```python
from build123d import *

# Parameters (mm, degrees)
F0_W     = 1
F0_H     = 2.4
F1_DEPTH = 10


# Not quite as in the source:
# - a feature names something its author has since deleted; it is built from what else it names


with BuildPart() as f1:
    # F0 (on Top) → F1 (new body)
    with BuildSketch(Plane.XY):
        with Locations((10.9311291858, -6.7)):
            Rectangle(F0_W, F0_H)
        with Locations((-10.6688708142, -6.7)):
            Rectangle(F0_W, F0_H)
        Polygon((-2.45, -8.5), (-2.45, -7.9), (-3.85, -7.9), (-1.45, -10.5), (-1.45, -8.5), align=None)
        with BuildLine():
            Line((-11.1688708142, -5.5), (-10.1688708142, -5.5))
            Line((-10.1688708142, -5.5), (-10.1688708142, -4.6410811281))
            ThreePointArc((-10.1688708142, -4.6410811281), (-10.8661281522, -4.8408828578), (-11.1688708142, -5.5))
        make_face()
        with BuildLine():
            Line((10.4311291858, -4.5), (10.4311291858, -5.5))
            Line((10.4311291858, -5.5), (11.4311291858, -5.5))
            ThreePointArc((11.4311291858, -5.5), (11.1382359669, -4.7928932188), (10.4311291858, -4.5))
        make_face()
        Polygon((-1.45, -5.5), (-2.45, -5.5), (-2.45, -7.9), (-2.45, -8.5), (-1.45, -8.5), align=None)
        Polygon((2.45, -5.5), (1.45, -5.5), (1.45, -8.5), (2.45, -8.5), (2.45, -7.9), align=None)
        with BuildLine():
            Line((-10.1688708142, -4.6410811281), (-10.1688708142, -5.5))
            Line((-10.1688708142, -5.5), (-2.45, -5.5))
            Line((-2.45, -5.5), (-1.45, -5.5))
            Line((-1.45, -5.5), (1.45, -5.5))
            Line((1.45, -5.5), (2.45, -5.5))
            Line((2.45, -5.5), (10.4311291858, -5.5))
            Line((10.4311291858, -5.5), (10.4311291858, -4.5))
            Line((10.4311291858, -4.5), (8.1, -4.5))
            ThreePointArc((8.1, -4.5), (4.5644660941, -3.0355339059), (3.1, 0.5))
            Line((3.1, 0.5), (3.1, 4))
            ThreePointArc((3.1, 4), (2.6606601718, 5.0606601718), (1.6, 5.5))
            Line((1.6, 5.5), (1.1, 5.5))
            Line((1.1, 5.5), (1.1, -4))
            Line((1.1, -4), (-1.1, -4))
            Line((-1.1, -4), (-1.1, 5.5))
            Line((-1.1, 5.5), (-1.6, 5.5))
            ThreePointArc((-1.6, 5.5), (-2.6606601718, 5.0606601718), (-3.1, 4))
            Line((-3.1, 4), (-3.1, 0.3589188719))
            ThreePointArc((-3.1, 0.3589188719), (-4.5644660941, -3.176615034), (-8.1, -4.6410811281))
            Line((-8.1, -4.6410811281), (-10.1688708142, -4.6410811281))
        make_face()
        Polygon((2.45, -8.5), (1.45, -8.5), (1.45, -10.5), (3.85, -7.9), (2.45, -7.9), align=None)
    extrude(amount=F1_DEPTH)


solid = f1.part
```
Source: CAD feature listing. Evaluate the final solid. Frame: model axes, mm. A direction names the side the tool comes from. Round coordinates to 2 decimals unless told otherwise and drop trailing zeros. Loops run counter-clockwise (first coordinate to the right, second up) from the corner with the lowest first, then second, coordinate; pieces in that order, holes last.
1. Contact query for flat-ended pins moving along their axis: pin 1 (1.9 mm diameter, centred on x = 9, z = 3, fed in from +Y); pin 2 (1.8 mm diameter, centred on y = 1.5, z = 3, fed in from -X); pin 3 (6 mm diameter, centred on x = 6.5, z = 1.5, fed in from +Y). Output: stop coordinate, or through.
2. Mould query, pull axis X, two halves, no side actions, for faces 6 (the flat face through (-1.45, -8, 5)), 7 (the flat face through (-11, -7.9, 5)), 8 (the cylindrical face through (4.6, -3.07, 4.93)). Classes: released by +X, released by -X, zero draft, split by the parting line, or undercut.
3. Section query A-A on y = 2. Output: boundary loops of the cut face in (x, z).
4. Ray query, L1, parallel to X at y = -5.75, z = 9.5; L2, parallel to X at y = 0.25, z = 5.5; L3, parallel to Y at x = 0.5, z = 3. Return the intervals inside material, ascending.
5. Section query C-C on x = -0.5. Output: boundary loops of the cut face in (y, z).
6. Section query D-D on y = -3.75. Output: boundary loops of the cut face in (x, z).
7. Access query for faces 1 (the flat face through (-2.45, -7, 5)), 2 (the flat face through (9, -4.5, 5)), 3 (the flat face through (11, -7.9, 5)), 4 (the flat face through (1.1, 1, 5)), 5 (the flat face through (10.431, -7, 5)). Directions: +Z, -Z, +X, -X, +Y, -Y. A direction counts if a zero-diameter tool reaches every point of the face in a straight line with its end or side. Return the directions, or none.
Answers below:
1. pin 1: stops at y = -4.5
1. pin 2: stops at x = -3.1
1. pin 3: stops at y = -1.46
2. face 6: undercut
2. face 7: zero draft
2. face 8: released by +X
3. outline: (-3.1, 0) - (-1.1, 0) - (-1.1, 10) - (-3.1, 10) - close; (1.1, 0) - (3.1, 0) - (3.1, 10) - (1.1, 10) - close
4. L1: x = -11.17 to -10.17, -2.45 to -1.45, 1.45 to 2.45, 10.43 to 11.43
4. L2: x = -3.1 to -1.1, 1.1 to 3.11
4. L3: y = -5.5 to -4
5. outline: (-5.5, 0) - (-4, 0) - (-4, 10) - (-5.5, 10) - close
6. outline: (-5.25, 0) - (-1.1, 0) - (-1.1, 10) - (-5.25, 10) - close; (1.1, 0) - (5.47, 0) - (5.47, 10) - (1.1, 10) - close
7. face 1: +Z, -Z
7. face 2: +Z, -Z, +X, +Y
7. face 3: +Z, -Z, +X, -Y
7. face 4: +Z, -Z, +Y
7. face 5: +Z, -Z, -Y
